Source: CAD feature listing. Evaluate the final solid. Frame: model axes, mm. A direction names the side the tool comes from. Give positions to 0.01 mm unless a question says otherwise; leave off trailing zeros. Loops run counter-clockwise (first coordinate to the right, second up) from the corner with the lowest first, then second, coordinate; pieces in that order, holes last. Notation, with made-up numbers: (83.5, 53.25) -> (128.5, 53.25) arc R26 cw to (128.5, 70.25) -> close; hole circle Ø6 at (87.25, 34.5). An arc over 180 degrees is marked (long way). Return JSON: item names as keys, results as strings. Group by question number.
```python
from build123d import *

# Parameters (mm, degrees)
SKETCH1_W         = 152.4
SKETCH1_H         = 152.4
EXTRUDE1_DEPTH    = 6.35
SKETCH2_R         = 1.5875
EXTRUDE2_DEPTH    = 108.95
SKETCH3_OUTSIDE_W = 197.524
SKETCH3_OUTSIDE_H = 197.524
EXTRUDE3_DEPTH    = 108.95


with BuildPart() as part:
    # Sketch1 → Extrude1 (new body)
    with BuildSketch(Plane.XY):
        Rectangle(SKETCH1_W, SKETCH1_H)
    extrude(amount=EXTRUDE1_DEPTH)

    # Sketch2 → Extrude2 (cut, through all)
    with BuildSketch(Plane.XY.offset(6.35)):
        with Locations((-63.5, 0)):
            Circle(SKETCH2_R)
        with Locations((38.1, 58.65878735)):
            Circle(SKETCH2_R)
        with Locations((38.1, -58.65878735)):
            Circle(SKETCH2_R)
    extrude(amount=-EXTRUDE2_DEPTH, mode=Mode.SUBTRACT)

    # Sketch3 outside → Extrude3 (cut, through all)
    with BuildSketch(Plane.XY.offset(6.35)):
        Rectangle(SKETCH3_OUTSIDE_W, SKETCH3_OUTSIDE_H)
        Polygon((-76.2, 12.7), (31.75, 12.7), (31.75, 76.2), (44.45, 76.2), (44.45, 12.7), (76.2, 12.7), (76.2, -12.7), (44.45, -12.7), (44.45, -76.2), (31.75, -76.2), (31.75, -12.7), (-76.2, -12.7), align=None, mode=Mode.SUBTRACT)
    extrude(amount=-EXTRUDE3_DEPTH, mode=Mode.SUBTRACT)

    # Sketch5 → CSK for 1/4 Flat Head Socket Cap Screw1 (revolve, cut)
    with BuildSketch(Plane.YZ.offset(-21.59)):
        Polygon((0, 0), (0, 6.35), (3.3782, 6.35), (3.3782, 3.728390023), (6.61924, 0), align=None)
    revolve(axis=Axis((-21.59, 0, -6.35), (0, 0, 1)), mode=Mode.SUBTRACT)

    # Sketch7 → CSK for 1/4 Flat Head Socket Cap Screw2 (revolve, cut)
    with BuildSketch(Plane.YZ.offset(44.45)):
        Polygon((0, 0), (0, 6.35), (3.3782, 6.35), (3.3782, 3.728390023), (6.61924, 0), align=None)
    revolve(axis=Axis((44.45, 0, -6.35), (0, 0, 1)), mode=Mode.SUBTRACT)


solid = part.part
```
1) Contact query for flat-ended pins moving along their axis: P1, Ø3, axis at y = 51, z = 3, coming from the +X side; P2, Ø1.9, axis at x = -18.5, z = 3, coming from the +Y side; P3, Ø11, axis at x = 44.45, y = 0, coming from the -Z side. Output: stop coordinate, or through.
2) Cut plane C-C on y = 30.5. Return loops of the section in (x, z).
3) Cut plane A-A on x = -21.59. Return loops of the section in (y, z).
4) Mould query, pull axis Y, two halves, no side actions, for faces 1 (the face through (-18.29, -0.73, 5.02)), 2 (the face through (-18.094, -0.776, 3.495)), 3 (the face through (61, -12.7, 3)), 4 (the face through (44.45, 45, 3)). Classes: released by +Y, released by -Y, zero draft, split by the parting line, or undercut.
5) Material intervals for line 1 (Y direction, x = 38.1, z = 2.75); line 2 (Y direction, x = 39, z = 1.75); line 3 (Y direction, x = -59.5, z = 0.5), sorted ascending.
6) Reachability of faces 5 (the face through (-23, 12.7, 3)), 6 (the face through (44.45, -44, 3)), 7 (the face through (60, 12.7, 3)), 8 (the face through (-21, -12.7, 3)) from +Z, -Z, +X, -X, +Y, -Y: full face, straight path, thin tool, end or side. Return the list, or none.
7) Cut plane B-B on z = 2.5. Count the separate pieces of the cut face and the enclosed holes in it, then the cut area to 3 significant figures.
Calculated:
{
 "1": {"P1": "x = 44.45", "P2": "y = 12.7", "P3": "z = 1.29"},
 "2": {"outline": "(31.75, 0) -> (44.45, 0) -> (44.45, 6.35) -> (31.75, 6.35) -> close"},
 "3": {"outline": "(-12.7, 0) -> (-6.62, 0) -> (-3.38, 3.73) -> (-3.38, 6.35) -> (-12.7, 6.35) -> close; (3.38, 3.73) -> (6.62, 0) -> (12.7, 0) -> (12.7, 6.35) -> (3.38, 6.35) -> close"},
 "4": {"face 1": "undercut", "face 2": "undercut", "face 3": "released by -Y", "face 4": "zero draft"},
 "5": {"line 1": "-76.2 to -60.25, -57.07 to 57.07, 60.25 to 76.2", "line 2": "-76.2 to -59.97, -57.35 to 57.35, 59.97 to 76.2", "line 3": "-12.7 to 12.7"},
 "6": {"face 5": "+Z, -Z, -X, +Y", "face 6": "+Z, -Z, +X, -Y", "face 7": "+Z, -Z, +X, +Y", "face 8": "+Z, -Z, -X, -Y"},
 "7": {"separate pieces": "1", "enclosed holes": "5", "area": "5,340 mm2"}
}
